The listing builds one solid part. Answer for the finished solid, in the listing's coordinates (mm). A direction names the side the tool comes from. Round coordinates to 2 decimals unless told otherwise and drop trailing zeros. Write each loop counter-clockwise with the first axis right and the second up, starting at its lowest first coordinate (ties: lowest second). Pieces come first, ordered by that corner, then holes.
(1) The mould has two halves that part along Z. Classify faces 1 (the face through (0, 3, 12)), 2 (the face through (-2.53, 2.96, -13.79)), 3 (the face through (0.75, 3, 22)), 4 (the face through (0, 3, 17.5)): +Z half, -Z half, draft (parallel to the pull), parting line (faces both ways), or undercut.
(2) A cutting plane is placed at D-D, the plane x = 2. Give the vertices of the cut face in (y, z), and give its area (3 significant figures).
(3) A cutting plane is placed at B-B, the plane y = 4.5. Give the vertices of the cut face in (x, z), and give its area (3 significant figures).
(4) A cutting plane is placed at C-C, the plane x = 0. Give the vertices of the cut face in (y, z).
(5) Each of these flat-tipped pins is pushed along its axis until it touches: pin 1 Ø8 at (x, z) = (-0.5, 6) entering from -Y; pin 2 Ø7.5 at (x, z) = (0, -10.5) entering from -Y; pin 3 Ø2 at (x, z) = (5.5, 15) entering from +Y. Where does it stop, or does it pass through?
(6) For faces 5 (the face through (-0.1, 8, 7.8)), 6 (the face through (0.1, 8, 11.8)), 7 (the face through (-0.75, 3, 22)), determine the directions among +Z, -Z, +X, -X, +Y, -Y from which every point of the face is accessible in a straight line to the end or side of a thin tool.
(7) A cutting plane is placed at A-A, the plane z = 13.5. Give the vertices of the cut face in (x, y).
(8) Find the intervals of material crossed by probe 1 along X at (y, z) = (4.85, -10.5); probe 2 along X at (y, z) = (2.2, 13.5); probe 3 along Y at (x, z) = (5.5, -1), in increasing order.
from build123d import *

# Parameters (mm, degrees)
SKETCH1_W           = 15
SKETCH1_H           = 35
SKETCH1_R           = 4.15
SKETCH1_R_2         = 1.5
BOSS_EXTRUDE1_DEPTH = 6
BOSS_EXTRUDE2_DEPTH = 4
SKETCH3_W           = 6.75
SKETCH3_H           = 6
BOSS_EXTRUDE3_DEPTH = 10


with BuildPart() as part:
    # Sketch1 → Boss-Extrude1 (new body)
    with BuildSketch(Plane(origin=(0, 0, 0), x_dir=(1, 0, 0), z_dir=(0, 1, 0))):
        Rectangle(SKETCH1_W, SKETCH1_H)
        with Locations(Location((0, 10.5, 0), (0, 0, 270))):  # turned: the seam where the file's is
            Circle(SKETCH1_R, mode=Mode.SUBTRACT)
        with Locations(Location((0, -13.5, 0), (0, 0, 270))):  # turned: the seam where the file's is
            Circle(SKETCH1_R_2, mode=Mode.SUBTRACT)
    extrude(amount=BOSS_EXTRUDE1_DEPTH)

    # Sketch2 → Boss-Extrude2 (add)
    with BuildSketch(Plane(origin=(0, 6, 0), x_dir=(1, 0, 0), z_dir=(0, 1, 0))):
        with BuildLine():
            Line((-7.5, -11.365857851), (-7.5, -7.365857851))
            ThreePointArc((-7.5, -7.365857851), (0, -7.8), (7.5, -7.365857851))
            Line((7.5, -7.365857851), (7.5, -11.365857851))
            ThreePointArc((7.5, -11.365857851), (0, -11.8), (-7.5, -11.365857851))
        make_face()
    extrude(amount=BOSS_EXTRUDE2_DEPTH)

    # Sketch3 → Boss-Extrude3 (add)
    with BuildSketch(Plane.XY.offset(17.5)):
        with Locations((4.125, 3)):
            Rectangle(SKETCH3_W, SKETCH3_H)
        with Locations((-4.125, 3)):
            Rectangle(SKETCH3_W, SKETCH3_H)
    extrude(amount=BOSS_EXTRUDE3_DEPTH)


solid = part.part
Solutions:
1. face 1: undercut
1. face 2: undercut
1. face 3: draft
1. face 4: +Z half
2. outline: (0, -17.5) - (6, -17.5) - (6, -14.14) - (0, -14.14) - close; (0, -6.86) - (6, -6.86) - (6, 7.77) - (10, 7.77) - (10, 11.77) - (6, 11.77) - (6, 27.5) - (0, 27.5) - close
2. area: 242 mm2
3. outline: (-7.5, -17.5) - (7.5, -17.5) - (7.5, 27.5) - (0.75, 27.5) - (0.75, 17.5) - (-0.75, 17.5) - (-0.75, 27.5) - (-7.5, 27.5) - close; hole circle Ø8.3 at (0, -10.5); hole circle Ø3 at (0, 13.5)
3. area: 599 mm2
4. outline: (0, -17.5) - (6, -17.5) - (6, -14.65) - (0, -14.65) - close; (0, -6.35) - (6, -6.35) - (6, 7.8) - (10, 7.8) - (10, 11.8) - (6, 11.8) - (6, 12) - (0, 12) - close; (0, 15) - (6, 15) - (6, 17.5) - (0, 17.5) - close
5. pin 1: stops at y = 0
5. pin 2: passes through
5. pin 3: stops at y = 6
6. face 5: -Z, +Y
6. face 6: +Z, +Y
6. face 7: +Z, +Y, -Y
7. outline: (-7.5, 0) - (-1.5, 0) - (-1.5, 6) - (-7.5, 6) - close; (1.5, 0) - (7.5, 0) - (7.5, 6) - (1.5, 6) - close
8. probe 1: x = -7.5 to -4.15, 4.15 to 7.5
8. probe 2: x = -7.5 to -1.5, 1.5 to 7.5
8. probe 3: y = 0 to 6
